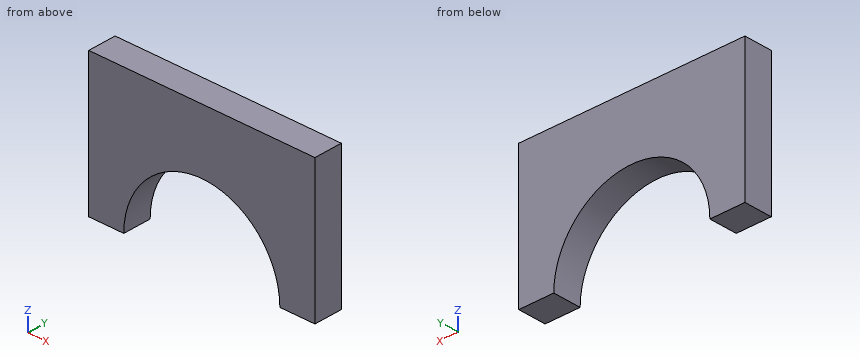
```python
from build123d import *

# Parameters (mm, degrees)
SKETCH1_W           = 50.8
SKETCH1_H           = 31.75
BOSS_EXTRUDE1_DEPTH = 6.35
CUT_EXTRUDE1_DEPTH  = 6.35


with BuildPart() as part:
    # Sketch1 → Boss-Extrude1 (new body)
    with BuildSketch(Plane(origin=(0, 0, 0), x_dir=(1, 0, 0), z_dir=(0, 1, 0))):
        Rectangle(SKETCH1_W, SKETCH1_H)
    extrude(amount=BOSS_EXTRUDE1_DEPTH)

    # Sketch2 → Cut-Extrude1 (cut)
    with BuildSketch(Plane(origin=(0, 6.35, 0), x_dir=(1, 0, 0), z_dir=(0, 1, 0))):
        with BuildLine():
            Line((-17.526, 15.875), (17.526, 15.875))
            ThreePointArc((17.526, 15.875), (0, -1.651), (-17.526, 15.875))
        make_face()
    extrude(amount=-CUT_EXTRUDE1_DEPTH, mode=Mode.SUBTRACT)


solid = part.part
```
Input: part model. Units: mm. Frame: model coordinates. Give positions to 0.01 mm unless a question says otherwise; leave off trailing zeros. Loops run counter-clockwise (first coordinate to the right, second up) from the corner with the lowest first, then second, coordinate; pieces in that order, holes last.
1) Contact query for a flat-ended pin moving along its axis: pin 1 (12 mm diameter, centred on x = -7.5, z = -11.5, fed in from -Y). Output: stop coordinate, or through.
A:
pin 1: passes through
2) Line query: L1, parallel to X at y = 1, z = -12; L2, parallel to X at y = 1.75, z = -12.5; L3, parallel to Z at x = -8, y = 2 (3 decimals). Output: solid intervals per line, ascending.
A:
L1: x = -25.4 to -17.09, 17.09 to 25.4
L2: x = -25.4 to -17.2, 17.2 to 25.4
L3: z = -0.281 to 15.875
3) Section query D-D on z = -11.5. Return the cut outline in (x, y).
A:
outline: (-25.4, 0) - (-16.97, 0) - (-16.97, 6.35) - (-25.4, 6.35) - close; (16.97, 0) - (25.4, 0) - (25.4, 6.35) - (16.97, 6.35) - close
4) Section query C-C on y = 3.5. Return the cut outline in (x, z) (3 decimals), and give its area (3 significant figures).
A:
outline: (-25.4, -15.875) - (-17.526, -15.875) arc R17.526 cw to (17.526, -15.875) - (25.4, -15.875) - (25.4, 15.875) - (-25.4, 15.875) - close
area: 1,130 mm2
5) Section query A-A on z = 1. Return the cut outline in (x, y), and give its area (3 significant figures).
A:
outline: (-25.4, 0) - (-4.73, 0) - (-4.73, 6.35) - (-25.4, 6.35) - close; (4.73, 0) - (25.4, 0) - (25.4, 6.35) - (4.73, 6.35) - close
area: 262 mm2
6) Section query B-B on x = 0. Return the cut outline in (y, z) (3 decimals), and give its area (3 significant figures).
A:
outline: (0, 1.651) - (6.35, 1.651) - (6.35, 15.875) - (0, 15.875) - close
area: 90.3 mm2
